from build123d import *

# Parameters (mm, degrees)
F0_W     = 69.85
F0_H     = 5.08
F1_DEPTH = 2.54
F2_R     = 2.53999
F4_D     = 3.81


# Not quite as in the source:
# - a fillet or chamfer is up to 0.001 mm smaller than in the source, because OpenCascade refuses the exact size


with BuildPart() as f1:
    # F0 (on Top) → F1 (new body)
    with BuildSketch(Plane.XY):
        with Locations((-40.0687940419, 48.9344280766)):
            Rectangle(F0_W, F0_H)
    extrude(amount=F1_DEPTH)

    # F2 (radius 2.54 in the source; OpenCascade refuses exactly that, so slightly less here)
    f2_edges = [f1.edges().sort_by_distance(p)[0] for p in [
        (-40.068794, 46.394428, 2.54),
        (-40.068794, 51.474428, 2.54),
    ]]
    fillet(f2_edges, radius=F2_R)

    # F4 (through all)
    with Locations(Plane.YZ.offset(-5.1437940419)):
        with Locations((48.9344280766, 0)):
            Hole(F4_D / 2)


solid = f1.part
Model file for the job. Use its own axes, mm. Coordinates: 2 decimals unless noted, no trailing zeros. Loops run counter-clockwise (first coordinate to the right, second up) from the corner with the lowest first, then second, coordinate; pieces in that order, holes last. Notation, with made-up numbers: (-10, 85) -> (24, 85) arc R22 ccw to (24, 101) -> close; hole circle Ø3 at (25.5, 11). An arc over 180 degrees is marked (long way). Use one line per item in the form item = value. Start each with the question number.
(1) Probe probe 1 along Y at (x, z) = (-39, 0.55); probe 2 along Y at (x, z) = (-31, 0.6); probe 3 along Z at (x, y) = (-63.5, 48.8). List the from-to ranges inside material, lowest first. Write a range as from..to.
(2) Flat gauge pin, fed straight in: pin 1 (1 mm diameter, centred on x = -25, z = 1.5, fed in from -Y). Where does the tip first touch, or does it go through?
(3) Pull direction Y, two halves, no side cores. Call faces 1 (the flat face through (-74.994, 48.7, 2.1)), 2 (the cylindrical face through (-40.558, 48.893, 1.905)), 3 (the cylindrical face through (-39.58, 47.12, 1.78)): pulls with the +Y half, pulls with the -Y half, needs draft (parallel to the pull), parting line crosses it, or undercut.
(4) Cut at A-A on z = 1.25. Give the cut face in (x, y), and give its area (3 significant figures).
(5) Cut at C-C on y = 47.9. Give the cut face in (x, z), and give its area (3 significant figures).
Values:
q1.probe_1 = 46.45..47.11, 50.76..51.41
q1.probe_2 = 46.47..47.13, 50.74..51.4
q1.probe_3 = 1.9..2.54
q2.pin_1 = 46.6
q3.face_1 = needs draft
q3.face_2 = undercut
q3.face_3 = pulls with the -Y half
q4.outline = (-74.99, 46.72) -> (-5.14, 46.72) -> (-5.14, 47.5) -> (-74.99, 47.5) -> close; (-74.99, 50.37) -> (-5.14, 50.37) -> (-5.14, 51.15) -> (-74.99, 51.15) -> close
q4.area = 108 mm2
q5.outline = (-74.99, 1.6) -> (-5.14, 1.6) -> (-5.14, 2.32) -> (-74.99, 2.32) -> close
q5.area = 50.3 mm2
